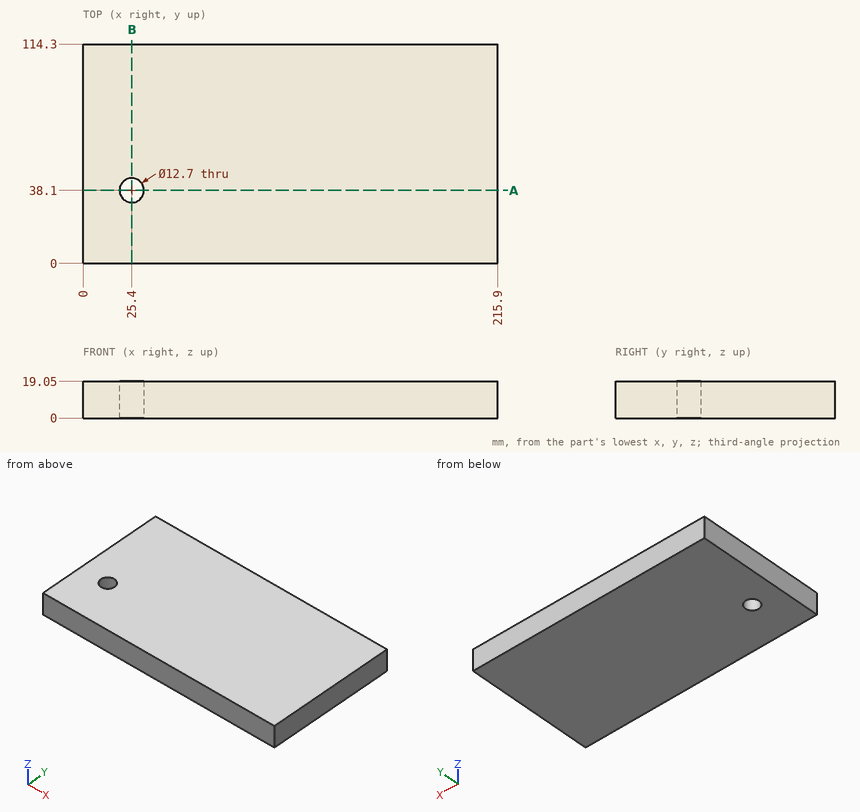
Input: dimensioned drawing with shaded views. Units: mm. Origin: part minimum x, y, z. Coordinates: 2 decimals unless noted, no trailing zeros. Order: outer loops, then holes, each group sorted by start corner. A loop starts at its lowest first (then second) coordinate and runs counter-clockwise, first axis right, second up. Notation, with made-up numbers: (65.25, -8.5) -> (98.25, -8.5) arc R15 cw to (98.25, 18.5) -> close; hole circle Ø10 at (5, -33). An arc over 180 degrees is marked (long way). Answer in a Markdown table with one row per item.
Item 1: Ray query, L1, parallel to X at y = 38.1, z = 9.5; L2, parallel to Y at x = 25.4, z = 13.25; L3, parallel to X at y = 34, z = 15. Return the intervals inside material, ascending.
Return value:
| item | result |
|---|---|
| L1 | x = 0 to 19.05, 31.75 to 215.9 |
| L2 | y = 0 to 31.75, 44.45 to 114.3 |
| L3 | x = 0 to 20.55, 30.25 to 215.9 |
Item 2: Section A-A on y = 38.1. Output: boundary loops of the cut face in (x, z).
Return value:
| item | result |
|---|---|
| outline | (0, 0) -> (19.05, 0) -> (19.05, 19.05) -> (0, 19.05) -> close; (31.75, 0) -> (215.9, 0) -> (215.9, 19.05) -> (31.75, 19.05) -> close |
Item 3: Section B-B on x = 25.4. Output: boundary loops of the cut face in (y, z).
Return value:
| item | result |
|---|---|
| outline | (0, 0) -> (31.75, 0) -> (31.75, 19.05) -> (0, 19.05) -> close; (44.45, 0) -> (114.3, 0) -> (114.3, 19.05) -> (44.45, 19.05) -> close |
